Model file for the job. Use its own axes, mm. Face numbers are marked on the shaded views. Round coordinates to 2 decimals unless told otherwise and drop trailing zeros. Order: outer loops, then holes, each group sorted by start corner. A loop starts at its lowest first (then second) coordinate and runs counter-clockwise, first axis right, second up. Notation, with made-up numbers: (-16, -17.75) - (12, -17.75) arc R18 cw to (12, 8.25) - close; hole circle Ø11 at (-12, 84). An arc over 180 degrees is marked (long way). Put each result on its own line as item: value. Start each with the question number.
Item 1: Saw through at A-A on z = -44. List the corners of the cut face in (x, y).
Item 2: Mould opens along Y. For the marked faces 1 and 2 say: pulls with the +Y half, pulls with the -Y half, needs draft (parallel to the pull), parting line crosses it, or undercut.
Item 3: Saw through at C-C on x = -23.5. List the corners of the cut face in (y, z), plus the area to 3 significant figures.
Item 4: Probe probe 1 along X at (y, z) = (0.7, -17); probe 2 along Z at (x, y) = (-15, 1.65); probe 3 along X at (y, z) = (1.65, -15.5). List the from-to ranges inside material, lowest first.
Item 5: Pin check, flat tips, straight feed: pin 1 Ø0.9 at (y, z) = (2, -9) entering from +X; pin 2 Ø5 at (x, z) = (59.5, -27.5) entering from -Y; pin 3 Ø1.5 at (x, y) = (-17, 2) entering from -Z; pin 4 Ø0.9 at (x, y) = (53.5, 1) entering from +Z. Stop position of each tip, or through.
Item 6: Saw through at D-D on y = 1.7. State how many separate pieces and enclosed holes the cut face has, plus the area to 3 significant figures.
Item 7: Saw through at B-B on x = 18. List the corners of the cut face in (y, z).
```python
from build123d import *

# Parameters (mm, degrees)
SKETCH_1_R          = 1.35
SKETCH_1_R_2        = 1.1
SKETCH_1_R_3        = 3.5
SKETCH_1_W          = 20
SKETCH_1_H          = 12
EXTRUDE_1_DEPTH     = 3
FILLET_1_R          = 5
SKETCH_2_R          = 1.6
CUT_EXTRUDE_1_DEPTH = 104.522944317
FILLET_2_R          = 2
SKETCH_4_R          = 1.5
CUT_EXTRUDE_3_DEPTH = 104.522944317


with BuildPart() as part:
    # 草图1 → 凸台-拉伸1 (new body)
    with BuildSketch(Plane(origin=(0, 0, 0), x_dir=(1, 0, 0), z_dir=(0, 1, 0))):
        Polygon((0, 0), (36, 0), (36, 24), (68, 24), (68, 29), (68, 53), (36, 53), (25, 59.350852961), (25, 78), (11, 78), (11, 59.350852961), (0, 53), (-32, 53), (-32, 29), (-32, 24), (0, 24), align=None)
        with Locations(Location((3, 3, 0), (0, 0, 270))):
            Circle(SKETCH_1_R, mode=Mode.SUBTRACT)
        with Locations(Location((3, 17, 0), (0, 0, 90))):
            Circle(SKETCH_1_R, mode=Mode.SUBTRACT)
        with Locations(Location((33, 3, 0), (0, 0, 90))):
            Circle(SKETCH_1_R, mode=Mode.SUBTRACT)
        with Locations(Location((33, 17, 0), (0, 0, 270))):
            Circle(SKETCH_1_R, mode=Mode.SUBTRACT)
        with Locations(Location((18, 74, 0), (0, 0, 270))):
            Circle(SKETCH_1_R_2, mode=Mode.SUBTRACT)
        with Locations(Location((18, 59, 0), (0, 0, 270))):
            Circle(SKETCH_1_R_2, mode=Mode.SUBTRACT)
        with Locations(Location((18, 44, 0), (0, 0, 270))):
            Circle(SKETCH_1_R_2, mode=Mode.SUBTRACT)
        with Locations(Location((18, 29, 0), (0, 0, 270))):
            Circle(SKETCH_1_R_2, mode=Mode.SUBTRACT)
        with Locations(Location((18, 36.5, 0), (0, 0, 270))):
            Circle(SKETCH_1_R_3, mode=Mode.SUBTRACT)
        with Locations((18, 9)):
            Rectangle(SKETCH_1_W, SKETCH_1_H, mode=Mode.SUBTRACT)
    extrude(amount=EXTRUDE_1_DEPTH)

    # 圆角1
    fillet_1_edges = [part.edges().sort_by_distance(p)[0] for p in [
        (11, 1.5, -78),
        (25, 1.5, -78),
        (25, 1.5, -59.350852961),
        (36, 1.5, -53),
        (68, 1.5, -53),
        (68, 1.5, -24),
        (36, 1.5, -24),
        (36, 1.5, 0),
        (0, 1.5, 0),
        (0, 1.5, -24),
        (-32, 1.5, -24),
        (-32, 1.5, -53),
        (0, 1.5, -53),
        (11, 1.5, -59.350852961),
    ]]
    fillet(fillet_1_edges, radius=FILLET_1_R)

    # 草图2 → 切除-拉伸1 (cut, through all)
    with BuildSketch(Plane(origin=(0, 3, 0), x_dir=(1, 0, 0), z_dir=(0, 1, 0))):
        with Locations(Location((5.5, 39.5, 0), (0, 0, 270))):
            Circle(SKETCH_2_R)
        with Locations(Location((5.5, 33.5, 0), (0, 0, 90))):
            Circle(SKETCH_2_R)
        with Locations(Location((30.5, 33.5, 0), (0, 0, 270))):
            Circle(SKETCH_2_R)
        with Locations(Location((30.5, 39.5, 0), (0, 0, 90))):
            Circle(SKETCH_2_R)
    extrude(amount=-CUT_EXTRUDE_1_DEPTH, mode=Mode.SUBTRACT)

    # 圆角2
    fillet_2_edges = [part.edges().sort_by_distance(p)[0] for p in [
        (28, 1.5, -3),
        (28, 1.5, -15),
        (8, 1.5, -15),
        (8, 1.5, -3),
    ]]
    fillet(fillet_2_edges, radius=FILLET_2_R)

    # 草图4 → 切除-拉伸3 (cut, through all)
    with BuildSketch(Plane(origin=(0, 3, 0), x_dir=(1, 0, 0), z_dir=(0, 1, 0))):
        with Locations(Location((-23.5, 37.5, 0), (0, 0, 270))):
            Circle(SKETCH_4_R)
        with Locations(Location((-23.5, 27.5, 0), (0, 0, 270))):
            Circle(SKETCH_4_R)
        with Locations(Location((-11.5, 37.5, 0), (0, 0, 270))):
            Circle(SKETCH_4_R)
        with Locations(Location((-11.5, 27.5, 0), (0, 0, 270))):
            Circle(SKETCH_4_R)
        with Locations(Location((47.5, 27.5, 0), (0, 0, 270))):
            Circle(SKETCH_4_R)
        with Locations(Location((47.5, 37.5, 0), (0, 0, 270))):
            Circle(SKETCH_4_R)
        with Locations(Location((59.5, 37.5, 0), (0, 0, 270))):
            Circle(SKETCH_4_R)
        with Locations(Location((59.5, 27.5, 0), (0, 0, 270))):
            Circle(SKETCH_4_R)
    extrude(amount=-CUT_EXTRUDE_3_DEPTH, mode=Mode.SUBTRACT)


solid = part.part
```
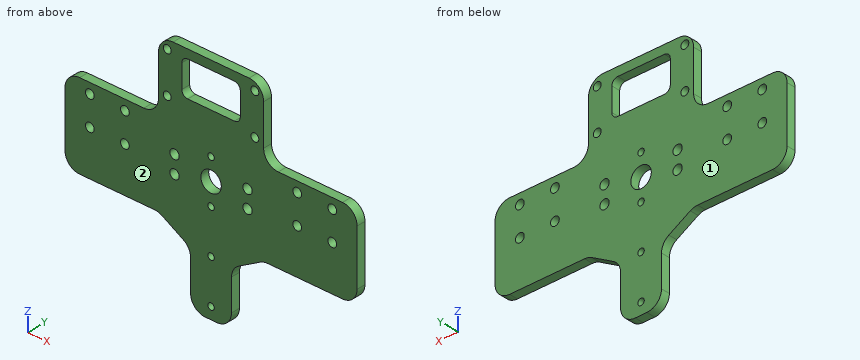
Results found:
1. outline: (-32, 0) - (16.9, 0) - (16.9, 3) - (-32, 3) - close; (19.1, 0) - (68, 0) - (68, 3) - (19.1, 3) - close
2. face 1: pulls with the +Y half
2. face 2: pulls with the -Y half
3. outline: (0, -53) - (3, -53) - (3, -39) - (0, -39) - close; (0, -36) - (3, -36) - (3, -29) - (0, -29) - close; (0, -26) - (3, -26) - (3, -24) - (0, -24) - close
3. area: 69.0 mm²
4. probe 1: x = 0 to 1.65, 4.35 to 31.65, 34.35 to 36
4. probe 2: z = -53 to -24
4. probe 3: x = 0 to 36
5. pin 1: stops at x = 36
5. pin 2: stops at y = 0
5. pin 3: stops at z = -53
5. pin 4: stops at z = -24
6. separate pieces: 1
6. enclosed holes: 22
6. area: 3,750 mm²
7. outline: (0, -78) - (3, -78) - (3, -75.1) - (0, -75.1) - close; (0, -72.9) - (3, -72.9) - (3, -60.1) - (0, -60.1) - close; (0, -57.9) - (3, -57.9) - (3, -45.1) - (0, -45.1) - close; (0, -42.9) - (3, -42.9) - (3, -40) - (0, -40) - close; (0, -33) - (3, -33) - (3, -30.1) - (0, -30.1) - close; (0, -27.9) - (3, -27.9) - (3, -15) - (0, -15) - close; (0, -3) - (3, -3) - (3, 0) - (0, 0) - close
